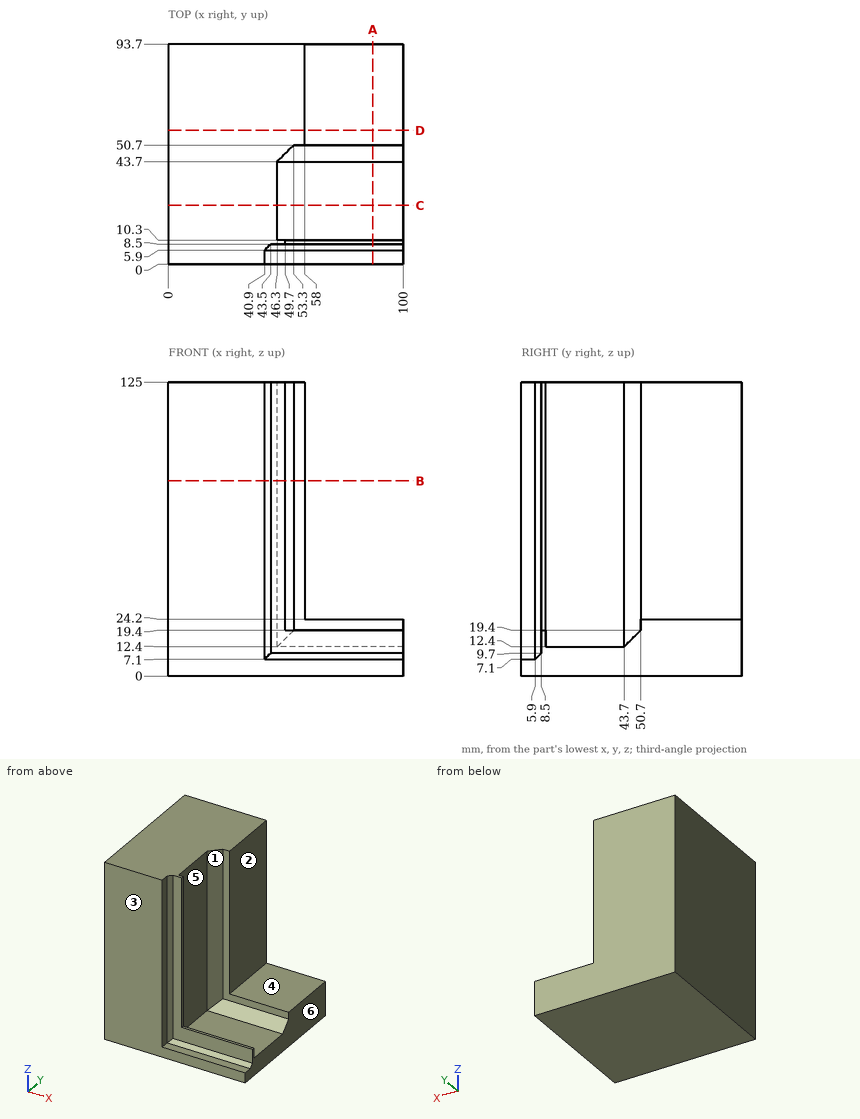
Job drawing, mm, ordinate dimensions from the low corner. One solid piece. A direction names the side the tool comes from. Round coordinates to 2 decimals unless told otherwise and drop trailing zeros. Order: outer loops, then holes, each group sorted by start corner. A loop starts at its lowest first (then second) coordinate and runs counter-clockwise, first axis right, second up. Notation, with made-up numbers: (46, -9.75) -> (69, -9.75) arc R24 cw to (69, 23.25) -> close; hole circle Ø4 at (-1, -2). An arc over 180 degrees is marked (long way). Answer in a Markdown table with one row per item.
1) Mould opens along Y. For the marked faces 1, 2 and 3 say: released by +Y, released by -Y, zero draft, split by the parting line, or undercut.
Values:
| item | result |
|---|---|
| face 1 | undercut |
| face 2 | zero draft |
| face 3 | released by -Y |
2) Pin check, flat tips, straight feed: P1, Ø10, axis at x = 66.5, y = 21, coming from the +Z side; P2, Ø3, axis at y = 3, z = 60, coming from the +X side; P3, Ø21, axis at x = 80.5, y = 65, coming from the +Z side. Stop position of each tip, or through.
Values:
| item | result |
|---|---|
| P1 | z = 12.4 |
| P2 | x = 40.9 |
| P3 | z = 24.2 |
3) Band-saw the part on C-C on y = 25. Give the cut face in (x, z), and give its area (3 significant figures).
Values:
| item | result |
|---|---|
| outline | (0, 0) -> (100, 0) -> (100, 12.4) -> (46.3, 12.4) -> (46.3, 125) -> (0, 125) -> close |
| area | 6,450 mm2 |
4) Which spindle directions (+Z, -Z, +X, -X, +Y, -Y) get a long thin tool onto all of the face, cutting with end or side? Do the marked faces 4, 5 and 6. Say none if no direction does.
Values:
| item | result |
|---|---|
| face 4 | +Z, +X, +Y, -Y |
| face 5 | +Z, +X |
| face 6 | +Z, -Z, +X, +Y, -Y |
5) Band-saw the part on D-D on y = 57. Give the cut face in (x, z), and give its area (3 significant figures).
Values:
| item | result |
|---|---|
| outline | (0, 0) -> (100, 0) -> (100, 24.2) -> (58, 24.2) -> (58, 125) -> (0, 125) -> close |
| area | 8,270 mm2 |
6) Band-saw the part on A-A on x = 87. Give the cut face in (y, z), and give its area (3 significant figures).
Values:
| item | result |
|---|---|
| outline | (0, 0) -> (93.7, 0) -> (93.7, 24.2) -> (50.7, 24.2) -> (50.7, 19.4) -> (43.7, 12.4) -> (10.3, 12.4) -> (10.3, 19.4) -> (8.5, 19.4) -> (8.5, 9.7) -> (5.9, 7.1) -> (0, 7.1) -> close |
| area | 1,660 mm2 |
7) Band-saw the part on B-B on z = 83. Give the cut face in (x, y), and give its area (3 significant figures).
Values:
| item | result |
|---|---|
| outline | (0, 0) -> (40.9, 0) -> (40.9, 5.9) -> (43.5, 8.5) -> (49.7, 8.5) -> (49.7, 10.3) -> (46.3, 10.3) -> (46.3, 43.7) -> (53.3, 50.7) -> (58, 50.7) -> (58, 93.7) -> (0, 93.7) -> close |
| area | 4,830 mm2 |
8) Wall check: L1, parallel to Z at x = 65, y = 67; L2, parallel to X at y = 40.5, z = 118.5; L3, parallel to Y at x = 57.5, z = 119.5. Give the ranges that are in metal, low to high.
Values:
| item | result |
|---|---|
| L1 | 0 to 24.2 |
| L2 | 0 to 46.3 |
| L3 | 50.7 to 93.7 |
